Source: CAD feature listing. Evaluate the final solid. Frame: model axes, mm. A direction names the side the tool comes from. Round coordinates to 2 decimals unless told otherwise and drop trailing zeros. Write each loop counter-clockwise with the first axis right and the second up, starting at its lowest first coordinate (ties: lowest second). Pieces come first, ordered by that corner, then holes. Notation, with made-up numbers: M 39,-33 L 67,-33 A28 ccw 67,4 Z; hole C 54.25,69 d8. An arc over 180 degrees is marked long. Use a Markdown table: item, result.
Autodesk Inventor part; units mm, degrees
ref_plane "YZ Plane" through (0, 0, 0) normal (1, 0, 0) x (0, 1, 0)
ref_plane "XZ Plane" through (0, 0, 0) normal (0, 1, 0) x (-1, 0, 0)
ref_plane "XY Plane" through (0, 0, 0) normal (0, 0, 1) x (1, 0, 0)
sketch "Эскиз1" plane through (0, 0, 0) normal (0, 1, 0) x (-1, 0, 0)
  line L0 (0, 0) -> (18.5, 0)
  line L1 (18.5, 0) -> (18.5, -16)
  line L2 (18.5, -16) -> (0, -16)
  line L3 (0, -16) -> (0, 0)
  dimension "d0" = 18.5
  dimension "d1" = 16
extrude "Выдавливание1" add sketch "Эскиз1" along normal blind 5
sketch "Эскиз2" plane through (0, 5, 0) normal (0, 1, 0) x (1, 0, 0)
  line L0 (-18.5, 16) -> (-18.5, 0)
  line L1 (-18.5, 8) -> (-12.5, 8)
  circle A0 centre (-12.5, 8) radius 4
  point P0 (0, 0)
  dimension "d4" = 6
  dimension "d5" = 8
extrude "Выдавливание2" cut sketch "Эскиз2" against normal blind 3
fillet "Сопряжение1" radius 8 2 edges at (-18.5, 2.5, 0) (-18.5, 2.5, -16)
sketch "Эскиз3" plane through (0, 0, 0) normal (0, -1, 0) x (1, 0, 0)
  line L0 (0, 0) -> (0, -16)
  line L1 (0, -8) -> (-2.5, -8)
  line L2 (-2.5, -3.5) -> (-2.5, -12.5)
  dimension "d9" = 2.5
  dimension "d10" = 9
hole "Отверстие1" at (-2.5, 0, -3.5) at (-2.5, 0, -12.5) direction (0, 1, 0) diameter 2.2 end through all countersink diameter 4.5 countersink angle 90
sketch "Эскиз4" plane through (0, 5, 0) normal (0, 1, 0) x (1, 0, 0)
  line L0 (0, 0) -> (-5, 0)
  line L1 (-5, 0) -> (-5, 16)
  line L2 (-5, 16) -> (0, 16)
  line L3 (0, 16) -> (0, 0)
  line L4 (0, 16) -> (-10.5, 16)
  dimension "d18" = 5
extrude "Выдавливание3" cut sketch "Эскиз4" against normal blind 1
properties part number "Деталь основы рулевого управления"
Q1. Section D-D on z = -7.25. Return loops of the section in (x, y), plus the area to 3 significant figures.
Results are:
| item | result |
|---|---|
| outline | M -18.46,0 L 0,0 L 0,4 L -5,4 L -5,5 L -8.57,5 L -8.57,2 L -16.43,2 L -16.43,5 L -18.46,5 Z |
| area | 63.7 mm^2 |
Q2. First-contact query: pin 1 Ø2.5 at (x, z) = (-14.5, -6.5) entering from +Y; pin 2 Ø0.5 at (y, z) = (4.5, -4) entering from +X; pin 3 Ø3 at (x, z) = (-2.5, -12.5) entering from -Y; pin 4 Ø1.3 at (x, z) = (-2.5, -3.5) entering from +Y. Flat tips, straight axial feed; report the tip coordinate or a pass-through.
Results are:
| item | result |
|---|---|
| pin 1 | y = 2 |
| pin 2 | x = -5 |
| pin 3 | y = 0.75 |
| pin 4 | through |
Q3. Reachability of faces 4 (the cylindrical face through (-13.367, 3.521, -4.095)), 5 (the flat face through (-5, 4.5, -7.9)), 6 (the cylindrical face through (-2.079, 2.595, -4.516)) from +Z, -Z, +X, -X, +Y, -Y: full face, straight path, thin tool, end or side. Return the list, or none.
Results are:
| item | result |
|---|---|
| face 4 | +Y |
| face 5 | +Z, -Z, +X, +Y |
| face 6 | +Y, -Y |
Q4. Section B-B on x = -2.5. Return loops of the section in (y, z).
Results are:
| item | result |
|---|---|
| outline | M 0,-16 L 4,-16 L 4,-13.6 L 1.15,-13.6 L 0,-14.75 Z; M 0,-10.25 L 1.15,-11.4 L 4,-11.4 L 4,-4.6 L 1.15,-4.6 L 0,-5.75 Z; M 0,-1.25 L 1.15,-2.4 L 4,-2.4 L 4,0 L 0,0 Z |
Q5. Line query: L1, parallel to Z at x = -2.5, y = 3.35; L2, parallel to X at y = 2.9, z = -11.5; L3, parallel to Y at x = -10.5, z = -5.75. Output: solid intervals per line, ascending.
Results are:
| item | result |
|---|---|
| L1 | -16 to -13.6, -11.4 to -4.6, -2.4 to 0 |
| L2 | -17.69 to -14.44, -10.56 to -2.96, -2.04 to 0 |
| L3 | 0 to 2 |
Q6. Mould query, pull axis X, two halves, no side actions, for faces 1 (the cylindrical face through (-16.219, 2.535, -2.406)), 2 (the flat face through (-13, 2, -8)), 3 (the flat face through (0, 2, -8)). Classes: +X half, -X half, draft (parallel to the pull), parting line (faces both ways), or undercut.
Results are:
| item | result |
|---|---|
| face 1 | -X half |
| face 2 | undercut |
| face 3 | +X half |
Q7. Section C-C on z = -3.5. Return loops of the section in (x, y).
Results are:
| item | result |
|---|---|
| outline | M -17.11,0 L -4.75,0 L -3.6,1.15 L -3.6,4 L -5,4 L -5,5 L -17.11,5 Z; M -1.4,1.15 L -0.25,0 L 0,0 L 0,4 L -1.4,4 Z |
